from build123d import *

# Parameters (mm, degrees)
F1_DEPTH       = 44.45
F3_ANGLE_BACK  = 90
F3_ANGLE       = 180
F5_DEPTH       = 12.7
F7_W           = 19.1765794656
F7_H           = 20.32
F8_DEPTH       = 38.1
F9_W           = 68.8219781561
F9_H           = 15.6805519946
F10_DEPTH      = 6.35
F12_DEPTH      = 2.54
F14_DEPTH      = 44.451
F14_DEPTH_BACK = 44.451
F15_W          = 4.3561459895
F15_H          = 5.5247349744
F16_DEPTH      = 0.254
F17_W          = 30.8628306508
F17_H          = 5.9643723071
F17_W_2        = 2.8725753073
F17_H_2        = 3.9488319308
F18_DEPTH      = 6.35
F19_ANGLE_BACK = 70
F19_ANGLE      = 140
F21_DEPTH      = 44.4510001
F21_DEPTH_BACK = 44.4510001
F22_W          = 63.8522766531
F22_H          = 1.2669962529
F23_DEPTH      = 2.54


with BuildPart() as f1:
    # F0 (on Right) → F1 (new body, symmetric)
    with BuildSketch(Plane.YZ):
        Polygon((-146.6177896183, -5.0897085369), (-147.32, -30.48), (106.68, -30.48), (106.68, 0), (0, 0), (-19.1765794656, 20.32), (-85.2165794656, 20.32), (-106.68, 2.4324294841), align=None)
    extrude(amount=F1_DEPTH, both=True)

    # F2 (on Right) → F3 (revolve, cut)
    with BuildSketch(Plane.YZ, mode=Mode.PRIVATE) as f3_sk:
        Polygon((-106.68, 2.4324294841), (-62.3583516914, 39.37), (-179.07, 39.37), (-179.07, -11.2019648213), align=None)
    revolve(f3_sk.sketch.rotate(Axis((0, -6.35, 51.4768799767), (0, 0, -1)), -F3_ANGLE_BACK), axis=Axis((0, -6.35, 51.4768799767), (0, 0, -1)), revolution_arc=F3_ANGLE, mode=Mode.SUBTRACT)

    # F4 (on face) → F5 (cut)
    with BuildSketch(Plane.XY):
        with BuildLine():
            Line((-30.6413764298, 7.2046327405), (29.4640543103, 7.2046327405))
            ThreePointArc((29.4640543103, 7.2046327405), (33.9541823709, 9.0645046799), (35.8140543103, 13.5546327405))
            Line((35.8140543103, 13.5546327405), (35.8140543103, 96.6237889767))
            ThreePointArc((35.8140543103, 96.6237889767), (33.9541823709, 101.1139170372), (29.4640543103, 102.9737889767))
            Line((29.4640543103, 102.9737889767), (-30.6413764298, 102.9737889767))
            ThreePointArc((-30.6413764298, 102.9737889767), (-35.1315044903, 101.1139170372), (-36.9913764298, 96.6237889767))
            Line((-36.9913764298, 96.6237889767), (-36.9913764298, 13.5546327405))
            ThreePointArc((-36.9913764298, 13.5546327405), (-35.1315044903, 9.0645046799), (-30.6413764298, 7.2046327405))
        make_face()
    extrude(amount=-F5_DEPTH, mode=Mode.SUBTRACT)

    # F7 (on Right) → F8 (cut, symmetric)
    with BuildSketch(Plane.YZ):
        with Locations((-9.5882897328, 10.16)):
            Rectangle(F7_W, F7_H)
    extrude(amount=F8_DEPTH, both=True, mode=Mode.SUBTRACT)

    # F9 (on face) → F10 (cut)
    with BuildSketch(Plane(origin=(0, -19.1765794656, 0), x_dir=(-1, 0, 0), z_dir=(0, 1, 0))):
        with Locations((0.006010922, 9.7910461482)):
            Rectangle(F9_W, F9_H)
    extrude(amount=-F10_DEPTH, mode=Mode.SUBTRACT)

    # F11 (on face) → F12 (cut)
    with BuildSketch(Plane(origin=(0, 106.68, 0), x_dir=(-1, 0, 0), z_dir=(0, 1, 0))):
        with BuildLine():
            Line((-21.59, -3.6485542078), (-44.45, -3.6485542078))
            Line((-44.45, -3.6485542078), (-44.45, -9.9976139794))
            Line((-44.45, -9.9976139794), (-21.59, -9.9976139794))
            ThreePointArc((-21.59, -9.9976139794), (-21.0511846327, -9.7744293467), (-20.828, -9.2356139794))
            Line((-20.828, -9.2356139794), (-20.828, -4.4105542078))
            ThreePointArc((-20.828, -4.4105542078), (-21.0511846327, -3.8717388405), (-21.59, -3.6485542078))
        make_face()
        with BuildLine():
            Line((44.45, -9.9976139794), (44.45, -3.6485542078))
            Line((44.45, -3.6485542078), (21.59, -3.6485542078))
            ThreePointArc((21.59, -3.6485542078), (21.0511846327, -3.8717388405), (20.828, -4.4105542078))
            Line((20.828, -4.4105542078), (20.828, -9.2356139794))
            ThreePointArc((20.828, -9.2356139794), (21.0511846327, -9.7744293467), (21.59, -9.9976139794))
            Line((21.59, -9.9976139794), (44.45, -9.9976139794))
        make_face()
    extrude(amount=-F12_DEPTH, mode=Mode.SUBTRACT)

    # F13 (on Right) → F14 (cut, two sides)
    with BuildSketch(Plane.YZ) as f14_sk:
        Polygon((-88.2660076022, 0), (-45.9169372916, 0), (-45.9169372916, 18.3047242463), (-69.1584387047, 18.3047242463), align=None)
    extrude(amount=-F14_DEPTH, mode=Mode.SUBTRACT)
    extrude(f14_sk.sketch, amount=F14_DEPTH_BACK, mode=Mode.SUBTRACT)

    # F15 (on face) → F16 (cut)
    with BuildSketch(Plane(origin=(0, 106.68, 0), x_dir=(-1, 0, 0), z_dir=(0, 1, 0))):
        with Locations((0.0063270053, -7.1436325128)):
            Rectangle(F15_W, F15_H)
    extrude(amount=-F16_DEPTH, mode=Mode.SUBTRACT)

    # F17 (on face) → F18 (cut)
    with BuildSketch(Plane(origin=(0, -146.3650721201, 4.0479674412), x_dir=(1, 0, 0), z_dir=(0, -0.9996177741, 0.027646078))):
        with Locations((-29.0185846746, -17.8666524589)):
            Rectangle(F17_W, F17_H)
        with Locations((29.0185846746, -17.8666524589)):
            Rectangle(F17_W, F17_H)
        with Locations((0, -17.8110701963)):
            Rectangle(F17_W_2, F17_H_2)
        Polygon((-32.4309132993, -33.338483423), (31.4213633537, -33.338483423), (31.4213633537, -31.7079313099), (31.4213633537, -30.8274384588), (31.4213633537, -28.3163934946), (-32.4309132993, -28.3163934946), (-32.4309132993, -30.8274384588), (-32.4309132993, -31.7079313099), align=None)
    extrude(amount=-F18_DEPTH, mode=Mode.SUBTRACT)

    # F6 (on Right) → F19 (revolve, cut)
    with BuildSketch(Plane.YZ, mode=Mode.PRIVATE) as f19_sk:
        Polygon((-181.2299340963, -30.48), (-147.32, -30.48), (-146.1423057277, 12.1026812121), (-181.2299340963, 12.1026812121), align=None)
    revolve(f19_sk.sketch.rotate(Axis((0, -25.1088291407, 39.4888808951), (0, 0, -1)), -F19_ANGLE_BACK), axis=Axis((0, -25.1088291407, 39.4888808951), (0, 0, -1)), revolution_arc=F19_ANGLE, mode=Mode.SUBTRACT)

    # F20 (on Right) → F21 (cut, two sides)
    with BuildSketch(Plane.YZ) as f21_sk:
        with BuildLine():
            Line((-126.2498049921, -30.48), (-100.8498049921, -30.48))
            ThreePointArc((-100.8498049921, -30.48), (-113.5498049921, -17.78), (-126.2498049921, -30.48))
        make_face()
        with BuildLine():
            Line((43.18, -30.48), (68.58, -30.48))
            ThreePointArc((68.58, -30.48), (55.88, -17.78), (43.18, -30.48))
        make_face()
    extrude(amount=F21_DEPTH, mode=Mode.SUBTRACT)
    extrude(f21_sk.sketch, amount=-F21_DEPTH_BACK, mode=Mode.SUBTRACT)

    # F22 (on face) → F23 (join)
    with BuildSketch(Plane(origin=(0, -140.0174992543, 3.8724148458), x_dir=(1, 0, 0), z_dir=(0, -0.9996177741, 0.027646078))):
        with Locations((-0.5047749728, -30.8253852965)):
            Rectangle(F22_W, F22_H)
    extrude(amount=F23_DEPTH)


solid = f1.part
Source: CAD feature listing. Evaluate the final solid. Frame: model axes, mm. A direction names the side the tool comes from. Give positions to 0.01 mm unless a question says otherwise; leave off trailing zeros. Write each loop counter-clockwise with the first axis right and the second up, starting at its lowest first coordinate (ties: lowest second). Pieces come first, ordered by that corner, then holes. Notation, with made-up numbers: M -18.5,0.25 L -8.5,0.25 A13 ccw -8.5,14.25 Z; hole C 14.25,65.5 d5. An arc over 180 degrees is marked long. Return JSON: item names as keys, results as strings. Group by question number.
1) Ray query, L1, parallel to Z at x = 11, y = -67.5; L2, parallel to Y at x = -1, z = -11; L3, parallel to Y at x = 24.5, z = -21. Return the intervals inside material, ascending.
2) Draft query along Y for faces 1 (the face through (34.003, 101.064, -6.261)), 2 (the face through (1, 87, -30.48)), 3 (the face through (0.74, -121.93, -0.44)). Return one class per face: released by +Y, released by -Y, zero draft, split by the parting line, or undercut.
3) Cut plane A-A, the plane z = 5. Output: boundary loops of the cut face in (x, y).
4) Cut plane C-C, the plane y = 17. Output: boundary loops of the cut face in (x, z).
5) Set-up query: faces 4 (the face through (0, -25.527, 10)), 5 (the face through (-1, -45.917, 9)), 6 (the face through (1, -52, 20.32)), 7 (the face through (38.1, -14, 6)), 8 (the face through (-1, 56, -12.7)). Return all of +Z, -Z, +X, -X, +Y, -Y with unobstructed straight access to the full face (end or side cutting, diameter ignored); none if empty.
6) Cut plane B-B, the plane y = 55.88. Output: boundary loops of the cut face in (x, z), then the cut area to 3 significant figures.
7) First-contact query: pin 1 Ø2 at (y, z) = (105.5, -7.5) entering from +X; pin 2 Ø12 at (x, y) = (-0.5, -94.5) entering from +Z; pin 3 Ø0.8 at (x, y) = (37.5, 105) entering from +Z; pin 4 Ø12 at (y, z) = (49.5, 9) entering from -X. Flat tips, straight axial feed; report the tip coordinate or a pass-through.
Data:
{
 "1": {"L1": "z = -30.48 to 0, 18.3 to 20.32", "L2": "y = -146.78 to 7.2, 102.97 to 106.68", "L3": "y = -144.57 to -122, -105.1 to 47.43, 64.33 to 106.68"},
 "2": {"face 1": "undercut", "face 2": "zero draft", "face 3": "released by -Y"},
 "3": {"outline": "M -44.45,-92.85 A97.25 ccw 44.45,-92.85 L 44.45,-83.05 L -44.45,-83.05 Z; M -44.45,-45.92 L 44.45,-45.92 L 44.45,-4.72 L 38.1,-4.72 L 38.1,-19.18 L 34.4,-19.18 L 34.4,-25.53 L -34.42,-25.53 L -34.42,-19.18 L -38.1,-19.18 L -38.1,-4.72 L -44.45,-4.72 Z"},
 "4": {"outline": "M -44.45,-30.48 L 44.45,-30.48 L 44.45,0 L 35.81,0 L 35.81,-12.7 L -36.99,-12.7 L -36.99,0 L -44.45,0 Z"},
 "5": {"face 4": "+Y", "face 5": "+X, -X", "face 6": "+Z, +X, -X, +Y, -Y", "face 7": "+Z, +Y", "face 8": "+Z"},
 "6": {"outline": "M -44.45,-17.78 L 44.45,-17.78 L 44.45,0 L 35.81,0 L 35.81,-12.7 L -36.99,-12.7 L -36.99,0 L -44.45,0 Z", "area": "656 mm²"},
 "7": {"pin 1": "stops at x = 20.83", "pin 2": "stops at z = 17.58", "pin 3": "stops at z = 0", "pin 4": "passes through"}
}
